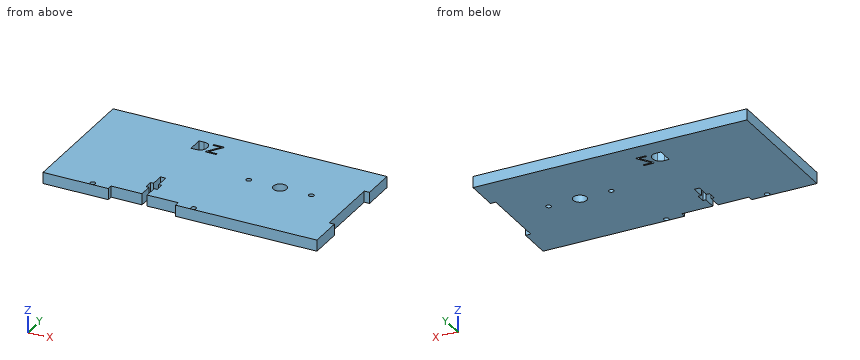
from build123d import *

# Parameters (mm, degrees)
F0_R     = 1.4605
F0_R_2   = 3.81
F1_DEPTH = 6.35


# Not quite as in the source:
# - a feature names something its author has since deleted; it is built from what else it names


with BuildPart() as f1:
    # F0 (on Top) → F1 (new body)
    with BuildSketch(Plane.XY):
        Polygon((72.9530500723, 9.1334713354), (72.9530500723, 28.1834713354), (-82.4187499277, 28.1834713354), (-82.4187499277, -48.0165286646), (-45.3947193277, -48.0165286646), (-45.3947193277, -45.0447286646), (-27.8052193277, -45.0447286646), (-27.8052193277, -37.4247286646), (-29.5197193277, -37.4247286646), (-29.5197193277, -32.4717286646), (-27.8052193277, -32.4717286646), (-27.8052193277, -24.8517286646), (-26.3447193277, -24.8517286646), (-24.8842193277, -24.8517286646), (-24.8842193277, -32.4717286646), (-23.1697193277, -32.4717286646), (-23.1697193277, -37.4247286646), (-24.8842193277, -37.4247286646), (-24.8842193277, -45.0447286646), (-7.2947193277, -45.0447286646), (-7.2947193277, -48.0165286646), (11.7552806723, -48.0165286646), (72.9530500723, -48.0165286646), (72.9530500723, -28.9665286646), (69.9812500723, -28.9665286646), (69.9812500723, 9.1334713354), align=None)
        with Locations((-54.9197193277, -46.5306286646)):
            Circle(F0_R, mode=Mode.SUBTRACT)
        with Locations((2.2302806723, -46.5306286646)):
            Circle(F0_R, mode=Mode.SUBTRACT)
        with BuildLine():
            add(Edge.make_bspline(
                [(-22.4210550397, 16.7985652577), (-21.283380549, 15.660890767), (-21.283380549, 13.6186639082)],
                knots=[0, 0, 0, 1, 1, 1], degree=2))
            add(Edge.make_bspline(
                [(-21.283380549, 13.6186639082), (-21.283380549, 11.4396463825), (-22.4663308238, 10.2865588589)],
                knots=[0, 0, 0, 1, 1, 1], degree=2))
            add(Edge.make_bspline(
                [(-22.4663308238, 10.2865588589), (-23.6492810986, 9.1334713354), (-25.8706844648, 9.1334713354)],
                knots=[0, 0, 0, 1, 1, 1], degree=2))
            Line((-25.8706844648, 9.1334713354), (-28.3097969206, 9.1334713354))
            Line((-28.3097969206, 9.1334713354), (-28.3097969206, 17.9362397483))
            Line((-28.3097969206, 17.9362397483), (-25.6125161638, 17.9362397483))
            add(Edge.make_bspline(
                [(-25.6125161638, 17.9362397483), (-23.5587295303, 17.9362397483), (-22.4210550397, 16.7985652577)],
                knots=[0, 0, 0, 1, 1, 1], degree=2))
        make_face(mode=Mode.SUBTRACT)
        Polygon((-13.9853094725, 10.0601799383), (-13.9853094725, 9.1334713354), (-20.0368515135, 9.1334713354), (-20.0368515135, 9.934949046), (-15.3647759168, 17.0153110328), (-19.8923543301, 17.0153110328), (-19.8923543301, 17.9362397483), (-14.1182468813, 17.9362397483), (-14.1182468813, 17.1347620377), (-18.790322478, 10.0601799383), align=None, mode=Mode.SUBTRACT)
        with Locations((12.9314999741, -7.1371421218)):
            Circle(F0_R, mode=Mode.SUBTRACT)
        with Locations((30.7114999741, -7.1371421218)):
            Circle(F0_R_2, mode=Mode.SUBTRACT)
        with Locations((48.4914999741, -7.1371421218)):
            Circle(F0_R, mode=Mode.SUBTRACT)
    extrude(amount=F1_DEPTH)


solid = f1.part
Part model, mm, in its own coordinate system. Coordinates: 2 decimals unless noted, no trailing zeros. Order: outer loops, then holes, each group sorted by start corner. A loop starts at its lowest first (then second) coordinate and runs counter-clockwise, first axis right, second up. Notation, with made-up numbers: M 52,-26.5 L 84,-26.5 A21 cw 84,-5.5 Z; hole C -24.75,-32.75 d5. An arc over 180 degrees is marked long. One line per question, with ' | ' between items.
Q1. Slice it at C-C (z = 5). Count the separate pieces of the cut face and the enclosed holes in it, and give its area (3 significant figures).
A:
separate pieces: 1 | enclosed holes: 7 | area: 11,400 mm^2
Q2. Slice it at B-B (y = 7). Give the cut face in (x, z).
A:
outline: M -82.42,0 L 69.98,0 L 69.98,6.35 L -82.42,6.35 Z
Q3. Slice it at A-A (x = 32). Give the cut face in (y, z), and give its area (3 significant figures).
A:
outline: M -48.02,0 L -10.72,0 L -10.72,6.35 L -48.02,6.35 Z; M -3.55,0 L 28.18,0 L 28.18,6.35 L -3.55,6.35 Z | area: 438 mm^2
Q4. Drill centre lines: line 1 (X direction, y = -37, z = 4.75); line 2 (X direction, y = -7.5, z = 4.75); line 3 (X direction, y = 11, z = 6.25). Where is each one in solid material? Low to high.
A:
line 1: x = -82.42 to -29.52, -23.17 to 72.95 | line 2: x = -82.42 to 11.52, 14.35 to 26.92, 34.5 to 47.08, 49.91 to 69.98 | line 3: x = -82.42 to -28.31, -21.9 to -19.33, -18.17 to 72.95
Q5. Pin check, flat tips, straight feed: P1, Ø3, axis at x = -18, z = 2, coming from the -Y side; P2, Ø1.9, axis at y = -13.5, z = 3, coming from the +X side; P3, Ø1.5, axis at x = -27, z = 4, coming from the -Y side. Stop position of each tip, or through.
A:
P1: stops at y = -45.04 | P2: stops at x = 69.98 | P3: stops at y = -24.85
Q6. Slice it at D-D (x = 48.5). Give the cut face in (y, z), and give its area (3 significant figures).
A:
outline: M -48.02,0 L -8.6,0 L -8.6,6.35 L -48.02,6.35 Z; M -5.68,0 L 28.18,0 L 28.18,6.35 L -5.68,6.35 Z | area: 465 mm^2
